Model file for the job. Use its own axes, mm. A direction names the side the tool comes from. Give positions to 0.01 mm unless a question says otherwise; leave off trailing zeros. Loops run counter-clockwise (first coordinate to the right, second up) from the corner with the lowest first, then second, coordinate; pieces in that order, holes last. Notation, with made-up numbers: (19.5, -35) - (38.5, -35) arc R11 cw to (38.5, -22) - close; hole circle Ø7 at (50, 10.25). An arc over 180 degrees is marked (long way). Use a Markdown table: item, result.
from build123d import *

# Parameters (mm, degrees)
F0_R     = 4.7625
F1_DEPTH = 18
F2_R     = 10.85
F2_R_2   = 4.7625
F3_DEPTH = 7
F4_R     = 1.5
F5_DEPTH = 12.5


with BuildPart() as f1:
    # F0 (on Top) → F1 (new body)
    with BuildSketch(Plane.XY):
        with BuildLine():
            Line((0, 10.85), (0, 9.85))
            ThreePointArc((0, 9.85), (-4.925, 8.53035), (-8.53035, 4.925))
            Line((-8.53035, 4.925), (-9.396376, 5.425))
            ThreePointArc((-9.396376, 5.425), (-10.85, 0), (-9.396376, -5.425))
            Line((-9.396376, -5.425), (-8.53035, -4.925))
            ThreePointArc((-8.53035, -4.925), (-4.925, -8.53035), (0, -9.85))
            Line((0, -9.85), (0, -10.85))
            ThreePointArc((0, -10.85), (5.425, -9.396376), (9.396376, -5.425))
            Line((9.396376, -5.425), (8.53035, -4.925))
            ThreePointArc((8.53035, -4.925), (9.85, 0), (8.53035, 4.925))
            Line((8.53035, 4.925), (9.396376, 5.425))
            ThreePointArc((9.396376, 5.425), (5.425, 9.396376), (0, 10.85))
        make_face()
        Circle(F0_R, mode=Mode.SUBTRACT)
    extrude(amount=F1_DEPTH)

    # F2 (on Top) → F3 (join)
    with BuildSketch(Plane.XY):
        Circle(F2_R)
        Circle(F2_R_2, mode=Mode.SUBTRACT)
    extrude(amount=F3_DEPTH)

    # F4 (on Front) → F5 (cut, symmetric)
    with BuildSketch(Plane.XZ):
        with Locations((0, 3.7)):
            Circle(F4_R)
    extrude(amount=F5_DEPTH, both=True, mode=Mode.SUBTRACT)


solid = f1.part
(1) Mould opens along Z. For faces 1 (the cylindrical face through (-0.195, 7.637, 5.187)), 2 (the flat face through (5, -2, 0)), 3 (the flat face through (-8.957, 5.172, 12.423)), 4 (the flat face through (-1, 5, 18)) say: pulls with the +Z half, pulls with the -Z half, needs draft (parallel to the pull), parting line crosses it, or undercut.
Computed:
| item | result |
|---|---|
| face 1 | undercut |
| face 2 | pulls with the -Z half |
| face 3 | needs draft |
| face 4 | pulls with the +Z half |
(2) Slice it at A-A, the plane y = 0. Write the cut outline in (x, z), plus the area to 3 significant figures.
Computed:
| item | result |
|---|---|
| outline | (-10.85, 0) - (-4.76, 0) - (-4.76, 18) - (-10.85, 18) - close; (4.76, 0) - (10.85, 0) - (10.85, 7) - (9.85, 7) - (9.85, 18) - (4.76, 18) - close |
| area | 208 mm² |
(3) Slice it at C-C, the plane x = -3.75. Write the cut outline in (y, z), plus the area to 3 significant figures.
Computed:
| item | result |
|---|---|
| outline | (-10.18, 0) - (-2.94, 0) - (-2.94, 18) - (-9.11, 18) - (-9.11, 7) - (-10.18, 7) - close; (2.94, 0) - (10.18, 0) - (10.18, 7) - (9.11, 7) - (9.11, 18) - (2.94, 18) - close |
| area | 237 mm² |
(4) Pin check, flat tips, straight feed: P1, Ø2, axis at x = -4, z = 6, coming from the -Y side; P2, Ø4, axis at x = -4, z = 5.5, coming from the -Y side; P3, Ø8, axis at y = 5, z = 3.5, coming from the +X side. Stop position of each tip, or through.
Computed:
| item | result |
|---|---|
| P1 | y = -10.43 |
| P2 | y = -10.66 |
| P3 | x = 10.8 |
(5) Drill centre lines: probe 1 along Z at (x, y) = (0, 7.5); probe 2 along Y at (x, z) = (-2.5, 13); probe 3 along X at (y, z) = (0.5, 4). Where is each one in solid material? Low to high. Write a range as [from, to].
Computed:
| item | result |
|---|---|
| probe 1 | [0, 2.2], [5.2, 18] |
| probe 2 | [-9.53, -4.05], [4.05, 9.53] |
| probe 3 | [-10.84, -4.74], [4.74, 10.84] |
(6) 3-axis set-ups, long thin cutter, end or side, ignore diameter. For faces 5 (the flat face through (0, -10, 12)), 6 (the flat face through (-8.97, -5.18, 12.42)), 7 (the flat face through (10, 0, 7)), 8 (the flat face through (0, 10.4, 12.4)): which of +Z, -Z, +X, -X, +Y, -Y reach the whole face in a straight line?
Computed:
| item | result |
|---|---|
| face 5 | +Z, -X, -Y |
| face 6 | +Z, -Y |
| face 7 | +Z, +X |
| face 8 | +Z, -X, +Y |
